Geometry: final body of the model. Coordinates: model frame, mm. A direction names the side the tool comes from. Give positions to 0.01 mm unless a question says otherwise; leave off trailing zeros. Order: outer loops, then holes, each group sorted by start corner. A loop starts at its lowest first (then second) coordinate and runs counter-clockwise, first axis right, second up. Notation, with made-up numbers: (55, 15.25) -> (75, 15.25) arc R24 cw to (75, 36.25) -> close; hole circle Ø9 at (67, -33.75). An arc over 180 degrees is marked (long way). Write item = value, one per line.
```python
from build123d import *

# Parameters (mm, degrees)
SKETCH_1_W           = 161.815887324
SKETCH_1_H           = 76.02828169
EXTRUDE_1_DEPTH      = 10
FILLET_1_R           = 10
CUT_EXTRUDE_5_DEPTH  = 27
SKETCH_5_R           = 38.014140845
EXTRUDE_2_DEPTH      = 80
EXTRUDE_4_DEPTH      = 45
EXTRUDE_4_DEPTH_BACK = 45
CUT_EXTRUDE_6_DEPTH  = 119
SKETCH_11_R          = 28.263571039
CUT_EXTRUDE_8_DEPTH  = 70
SKETCH_12_R          = 14.431437431
CUT_EXTRUDE_9_DEPTH  = 70


with BuildPart() as part:
    # 草图1 → 凸台-拉伸1 (new body)
    with BuildSketch(Plane(origin=(0, 0, 0), x_dir=(1, 0, 0), z_dir=(0, 1, 0))):
        Rectangle(SKETCH_1_W, SKETCH_1_H)
    extrude(amount=EXTRUDE_1_DEPTH)

    # 圆角1
    fillet_1_edges = [part.edges().sort_by_distance(p)[0] for p in [
        (80.907943662, 5, 38.014140845),
        (-80.907943662, 5, 38.014140845),
        (-80.907943662, 5, -38.014140845),
        (80.907943662, 5, -38.014140845),
    ]]
    fillet(fillet_1_edges, radius=FILLET_1_R)

    # 草图4 → 切除-拉伸5 (cut)
    with BuildSketch(Plane(origin=(0, 0, 0), x_dir=(1, 0, 0), z_dir=(0, 1, 0))):
        with BuildLine():
            Line((-80.907943662, 7.242463814), (-64.523768529, 7.242463814))
            ThreePointArc((-64.523768529, 7.242463814), (-57.281304715, 0), (-64.523768529, -7.242463814))
            Line((-64.523768529, -7.242463814), (-80.907943662, -7.242463814))
            Line((-80.907943662, -7.242463814), (-80.907943662, 7.242463814))
        make_face()
    cut_extrude_5 = extrude(amount=CUT_EXTRUDE_5_DEPTH, mode=Mode.SUBTRACT)

    # 镜向7: 切除-拉伸5 across plane
    add(cut_extrude_5.mirror(Plane(origin=(0, 0, 0), x_dir=(0, 0, 1), z_dir=(1, 0, 0))), mode=Mode.SUBTRACT)

    # 草图5 → 凸台-拉伸2 (add)
    with BuildSketch(Plane(origin=(0, 0, 0), x_dir=(1, 0, 0), z_dir=(0, 1, 0))):
        with Locations(Location((0, 0, 0), (0, 0, 270))):
            Circle(SKETCH_5_R)
    extrude(amount=EXTRUDE_2_DEPTH)

    # 草图6 → 凸台-拉伸4 (add, two sides: drawn at the far end of the back side and taken through both)
    with BuildSketch(Plane.XY.offset(-EXTRUDE_4_DEPTH_BACK)):
        with BuildLine():
            Line((-12.762943226, 0), (-12.762943226, 48.559275417))
            ThreePointArc((-12.762943226, 48.559275417), (0, 61.322218643), (12.762943226, 48.559275417))
            Line((12.762943226, 48.559275417), (12.762943226, 0))
            Line((12.762943226, 0), (-12.762943226, 0))
        make_face()
    extrude(amount=EXTRUDE_4_DEPTH + EXTRUDE_4_DEPTH_BACK)

    # 草图9 → 切除-拉伸6 (cut)
    with BuildSketch(Plane.XY.offset(45)):
        with BuildLine():
            Line((-8.103456016, 0), (-8.103456016, 48.501805974))
            ThreePointArc((-8.103456016, 48.501805974), (0, 56.60526199), (8.103456016, 48.501805974))
            Line((8.103456016, 48.501805974), (8.103456016, 0))
            Line((8.103456016, 0), (-8.103456016, 0))
        make_face()
    extrude(amount=-CUT_EXTRUDE_6_DEPTH, mode=Mode.SUBTRACT)

    # 草图11 → 切除-拉伸8 (cut)
    with BuildSketch(Plane.XZ):
        with Locations(Location((0, 0, 0), (0, 0, 270))):
            Circle(SKETCH_11_R)
    extrude(amount=-CUT_EXTRUDE_8_DEPTH, mode=Mode.SUBTRACT)

    # 草图12 → 切除-拉伸9 (cut)
    with BuildSketch(Plane(origin=(0, 80, 0), x_dir=(1, 0, 0), z_dir=(0, 1, 0))):
        with Locations(Location((0, 0, 0), (0, 0, 270))):
            Circle(SKETCH_12_R)
    extrude(amount=-CUT_EXTRUDE_9_DEPTH, mode=Mode.SUBTRACT)


solid = part.part
```
1) First-contact query: P1, Ø11, axis at x = -76, y = 3, coming from the -Z side; P2, Ø17.5, axis at x = 0, z = 0, coming from the +Y side; P3, Ø4.5, axis at y = 24, z = 40, coming from the +X side; P4, Ø12, axis at x = -19.5, y = 21.5, coming from the -Z side. Flat tips, straight axial feed; report the tip coordinate or a pass-through.
Check sheet entries:
P1 = -38.01
P2 = through
P3 = 12.76
P4 = -35.54
2) Section query B-B (x = 0). Output: boundary loops of the cut face in (y, z), plus the area to 3 significant figures.
Check sheet entries:
outline = (56.61, -45) -> (61.32, -45) -> (61.32, -38.01) -> (80, -38.01) -> (80, -14.43) -> (70, -14.43) -> (70, -28.26) -> (56.61, -28.26) -> close; (56.61, 28.26) -> (70, 28.26) -> (70, 14.43) -> (80, 14.43) -> (80, 38.01) -> (61.32, 38.01) -> (61.32, 45) -> (56.61, 45) -> close
area = 799 mm²
3) Section query C-C (y = 73.5). Output: boundary loops of the cut face in (x, z), plus the area to 3 significant figures.
Check sheet entries:
outline = circle Ø76.03 at (0, 0); hole circle Ø28.86 at (0, 0)
area = 3,890 mm²
4) Reachability of faces 1 (the face through (-73, 5, 7.242)), 2 (the face through (13, 70, 7)), 3 (the face through (8.103, 25, 36)), 4 (the face through (-33.725, 44.51, 17.541)) from +Z, -Z, +X, -X, +Y, -Y: full face, straight path, thin tool, end or side. Return the list, or none.
Check sheet entries:
face_1 = -X, +Y, -Y
face_2 = -Y
face_3 = +Z, -Z, -Y
face_4 = +Y
5) Mould query, pull axis Y, two halves, no side actions, for faces 5 (the face through (-0.178, 56.603, -35.913)), 6 (the face through (-55, 10, -1)), 7 (the face through (73, 5, -7.242)). Classes: +Y half, -Y half, draft (parallel to the pull), parting line (faces both ways), or undercut.
Check sheet entries:
face_5 = -Y half
face_6 = +Y half
face_7 = draft
6) Section query D-D (z = 18). Output: boundary loops of the cut face in (x, y), plus the area to 3 significant figures.
Check sheet entries:
outline = (-80.91, 0) -> (-21.79, 0) -> (-21.79, 70) -> (21.79, 70) -> (21.79, 0) -> (80.91, 0) -> (80.91, 10) -> (33.48, 10) -> (33.48, 80) -> (-33.48, 80) -> (-33.48, 10) -> (-80.91, 10) -> close
area = 3,260 mm²
7) Section query A-A (y = 16.5). Output: boundary loops of the cut face in (x, z).
Check sheet entries:
outline = (-12.76, -45) -> (-8.1, -45) -> (-8.1, -27.08) arc R28.26 cw to (-8.1, 27.08) -> (-8.1, 45) -> (-12.76, 45) -> (-12.76, 35.81) arc R38.01 ccw to (-12.76, -35.81) -> close; (8.1, -45) -> (12.76, -45) -> (12.76, -35.81) arc R38.01 ccw to (12.76, 35.81) -> (12.76, 45) -> (8.1, 45) -> (8.1, 27.08) arc R28.26 cw to (8.1, -27.08) -> close
8) Line query: line 1 (X direction, y = 13.5, z = 39.5); line 2 (X direction, y = 45, z = 0); line 3 (Y direction, x = -46.5, z = -21.5). Output: solid intervals per line, ascending. Write a range as from..to.
Check sheet entries:
line_1 = -12.76..-8.1, 8.1..12.76
line_2 = -38.01..-28.26, 28.26..38.01
line_3 = 0..10
